```python
from build123d import *

# Parameters (mm, degrees)
F1_DEPTH = 120
F2_SIZE  = 19.99999
F3_R     = 1.5
F4_DEPTH = 20.001


# Not quite as in the source:
# - a fillet or chamfer is up to 0.001 mm smaller than in the source, because OpenCascade refuses the exact size


with BuildPart() as f1:
    # F0 (on Front) → F1 (new body, symmetric)
    with BuildSketch(Plane.XZ):
        Polygon((-2, 0), (0, 0), (0, 20), (-20, 20), (-20, 18), (-2, 18), align=None)
    extrude(amount=F1_DEPTH, both=True)

    # F2 (size 20 in the source; OpenCascade refuses exactly that, so slightly less here)
    f2_edges = [f1.edges().sort_by_distance(p)[0] for p in [
        (-20, -120, 19),
        (-20, 120, 19),
    ]]
    chamfer(f2_edges, length=F2_SIZE)

    # F3 (on face) → F4 (cut, through all)
    with BuildSketch(Plane.YZ):
        with Locations((111, 10)):
            Circle(F3_R)
        with Locations((-111, 10)):
            Circle(F3_R)
    extrude(amount=-F4_DEPTH, mode=Mode.SUBTRACT)


solid = f1.part
```
For this review, take the finished solid that the model builds, in its own axes (mm). A direction names the side the tool comes from. Round coordinates to 2 decimals unless told otherwise and drop trailing zeros. Write each loop counter-clockwise with the first axis right and the second up, starting at its lowest first coordinate (ties: lowest second). Pieces come first, ordered by that corner, then holes. Notation, with made-up numbers: (25.25, 89) - (61.25, 89) arc R23 cw to (61.25, 124) - close; hole circle Ø5 at (12, 28). An arc over 180 degrees is marked (long way). Answer as CSV lines item,"result". Start each with the question number.
(1) For pin 1 (1.8 mm diameter, centred on y = 111, z = 10, fed in from -X); pin 2 (10 mm diameter, centred on y = -42.5, z = 8, fed in from +X); pin 3 (5.5 mm diameter, centred on y = 58, z = 4.5, fed in from -X); pin 4 (3 mm diameter, centred on x = -9.5, y = -11, fed in from -Z), all flat-tipped, find the tip position at first contact; note any pin that passes through.
(2) Add section B-B, the plane x = -15.5. State the section outline as (y, z) points, plus the area to 3 significant figures.
(3) Add section C-C, the plane x = -5.5. State the section outline as (y, z) points, plus the area to 3 significant figures.
(4) For line 1 (Z direction, x = -0.8, y = 111); line 2 (X direction, y = -107, z = 6.75); line 3 (Z direction, x = -15.5, y = 37), list the stretches that pass through material, from the lowest coordinate up.
(5) Add section A-A, the plane y = -37.5. State the section outline as (x, z) points.
(6) Mouldability with a two-part tool opening along X and no side actions: class faces 1 (the flat face through (-5.5, -114.5, 18.2)), 2 (the flat face through (-11, -2, 18)), 3 (the flat face through (0, -2, 10)) as +X half, -X half, draft (parallel to the pull), parting line (faces both ways), or undercut.
(7) Machinability: for faces 4 (the flat face through (-2, -2, 9)), 5 (the flat face through (-5.5, 114.5, 18.2)), which of the approach directions +Z, -Z, +X, -X, +Y, -Y give a long, thin tool a straight path to every point of the face, cutting with its end or side? Answer none if there is none.
From the geometry:
1,pin 1,"passes through"
1,pin 2,"stops at x = 0"
1,pin 3,"stops at x = -2"
1,pin 4,"stops at z = 18"
2,outline,"(-104.5, 18) - (104.5, 18) - (104.5, 20) - (-104.5, 20) - close"
2,area,"418 mm²"
3,outline,"(-114.5, 18) - (114.5, 18) - (114.5, 20) - (-114.5, 20) - close"
3,area,"458 mm²"
4,line 1,"z = 0 to 8.5, 11.5 to 20"
4,line 2,"x = -2 to 0"
4,line 3,"z = 18 to 20"
5,outline,"(-20, 18) - (-2, 18) - (-2, 0) - (0, 0) - (0, 20) - (-20, 20) - close"
6,face 1,"-X half"
6,face 2,"draft"
6,face 3,"+X half"
7,face 4,"-Z, -X, +Y, -Y"
7,face 5,"+Z, -Z, -X, +Y"
